from build123d import *

# Parameters (mm, degrees)
BOSS_EXTRUDE1_DEPTH = 6
SKETCH2_W           = 80
SKETCH2_H           = 80
CUT_EXTRUDE1_DEPTH  = 6
SKETCH3_W           = 60
SKETCH3_H           = 60
CUT_EXTRUDE2_DEPTH  = 6
CUT_EXTRUDE3_DEPTH  = 10
SKETCH6_W           = 40
SKETCH6_H           = 43
CUT_EXTRUDE4_DEPTH  = 7
SKETCH7_W           = 6
SKETCH7_H           = 15
CUT_EXTRUDE5_DEPTH  = 7


with BuildPart() as part:
    # Sketch1 → Boss-Extrude1 (new body)
    with BuildSketch(Plane(origin=(0, 0, 0), x_dir=(0, 0, -1), z_dir=(1, 0, 0))):
        with BuildLine():
            Line((-125, -82.915619759), (125, -82.915619759))
            ThreePointArc((125, -82.915619759), (0, 150), (-125, -82.915619759))
        make_face()
    extrude(amount=BOSS_EXTRUDE1_DEPTH)

    # Sketch2 → Cut-Extrude1 (cut)
    with BuildSketch(Plane(origin=(6, 0, 0), x_dir=(0, 0, -1), z_dir=(1, 0, 0))):
        with Locations((-90, 0)):
            Rectangle(SKETCH2_W, SKETCH2_H)
        with Locations((90, 0)):
            Rectangle(SKETCH2_W, SKETCH2_H)
    extrude(amount=-CUT_EXTRUDE1_DEPTH, mode=Mode.SUBTRACT)

    # Sketch3 → Cut-Extrude2 (cut)
    with BuildSketch(Plane(origin=(6, 0, 0), x_dir=(0, 0, -1), z_dir=(1, 0, 0))):
        with Locations((0, 100)):
            Rectangle(SKETCH3_W, SKETCH3_H)
    extrude(amount=-CUT_EXTRUDE2_DEPTH, mode=Mode.SUBTRACT)

    # Sketch4 → Cut-Extrude3 (cut)
    with BuildSketch(Plane(origin=(6, 0, 0), x_dir=(0, 0, -1), z_dir=(1, 0, 0))):
        Polygon((-90, -40), (-84, -40), (-84, -46), (-41, -46), (-41, -40), (-35, -40), (-35, -54), (-41, -54), (-41, -60), (-80, -60), (-80, -54), (-90, -54), align=None)
        Polygon((-80, 60), (-41, 60), (-41, 54), (-35, 54), (-35, 40), (-41, 40), (-41, 46), (-84, 46), (-84, 40), (-90, 40), (-90, 54), (-80, 54), align=None)
        Polygon((80, -60), (41, -60), (41, -54), (35, -54), (35, -40), (41, -40), (41, -46), (84, -46), (84, -40), (90, -40), (90, -54), (80, -54), align=None)
        Polygon((90, 40), (90, 54), (80, 54), (80, 60), (41, 60), (41, 54), (35, 54), (35, 40), (41, 40), (41, 46), (84, 46), (84, 40), align=None)
    extrude(amount=-CUT_EXTRUDE3_DEPTH, mode=Mode.SUBTRACT)

    # Sketch6 → Cut-Extrude4 (cut, through all)
    with BuildSketch(Plane(origin=(6, 0, 0), x_dir=(0, 0, -1), z_dir=(1, 0, 0))):
        with Locations((-30, 0)):
            Rectangle(SKETCH6_W, SKETCH6_H)
        with Locations((30, 0)):
            Rectangle(SKETCH6_W, SKETCH6_H)
    extrude(amount=-CUT_EXTRUDE4_DEPTH, mode=Mode.SUBTRACT)

    # Sketch7 → Cut-Extrude5 (cut, through all)
    with BuildSketch(Plane(origin=(6, 0, 0), x_dir=(0, 0, -1), z_dir=(1, 0, 0))):
        with Locations((-33, 122.5)):
            Rectangle(SKETCH7_W, SKETCH7_H)
        with Locations((-33, 77.5)):
            Rectangle(SKETCH7_W, SKETCH7_H)
        with Locations((33, 77.5)):
            Rectangle(SKETCH7_W, SKETCH7_H)
        with Locations((33, 122.5)):
            Rectangle(SKETCH7_W, SKETCH7_H)
    extrude(amount=-CUT_EXTRUDE5_DEPTH, mode=Mode.SUBTRACT)


solid = part.part
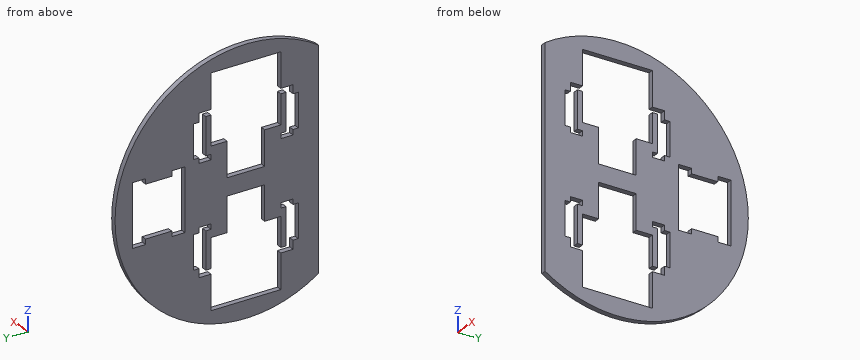
The listing builds one solid part. Answer for the finished solid, in the listing's coordinates (mm). Give positions to 0.01 mm unless a question says otherwise; leave off trailing zeros. Write each loop counter-clockwise with the first axis right and the second up, starting at its lowest first coordinate (ties: lowest second). Pieces come first, ordered by that corner, then holes.
Item 1: Section C-C, the plane y = 97 is taken. Write down the section's boundary in (x, z).
Item 2: Section B-B, the plane y = 0 is taken. Write down the section's boundary in (x, z).
Item 3: Find the intervals of material crossed by line 1 along Z through (x, y) = (3.6, -3); line 2 along Z through (x, y) = (3.8, 3.5); line 3 along Y through (x, z) = (4.35, -69.5), in increasing order.
Item 4: Flat-ended cylindrical pins translate along their axes: P1, Ø2, axis at x = 5, y = 47.5, coming from the -Z side; P2, Ø1.8, axis at x = 2.5, z = -34.5, coming from the +Y side; P3, Ø1.5, axis at x = 5, y = 22.5, coming from the +Z side. Find the tip coordinate at first contact, or state that the pin passes through.
Item 5: Section D-D, the plane z = 53.5 is taken. Write down the section's boundary in (x, y), plus the area to 3 significant figures.
Item 6: Section A-A, the plane z = 0 is taken. Write down the section's boundary in (x, y), plus the area to 3 significant figures.
Completed:
1. outline: (0, -114.42) - (6, -114.42) - (6, -30) - (0, -30) - close; (0, 30) - (6, 30) - (6, 114.42) - (0, 114.42) - close
2. outline: (0, -150) - (6, -150) - (6, -130) - (0, -130) - close; (0, -10) - (6, -10) - (6, 10) - (0, 10) - close; (0, 130) - (6, 130) - (6, 150) - (0, 150) - close
3. line 1: z = -149.97 to -130, -10 to 10, 130 to 149.97
3. line 2: z = -149.96 to -130, -10 to 10, 130 to 149.96
3. line 3: y = -82.92 to -60, -46 to -40, 40 to 46, 60 to 132.93
4. P1: stops at z = -142.61
4. P2: stops at y = 146.19
4. P3: stops at z = 148.41
5. outline: (0, -82.92) - (6, -82.92) - (6, -60) - (0, -60) - close; (0, -46) - (6, -46) - (6, -40) - (0, -40) - close; (0, 40) - (6, 40) - (6, 46) - (0, 46) - close; (0, 60) - (6, 60) - (6, 140.13) - (0, 140.13) - close
5. area: 690 mm2
6. outline: (0, -82.92) - (6, -82.92) - (6, 70) - (0, 70) - close; (0, 130) - (6, 130) - (6, 150) - (0, 150) - close
6. area: 1,040 mm2
